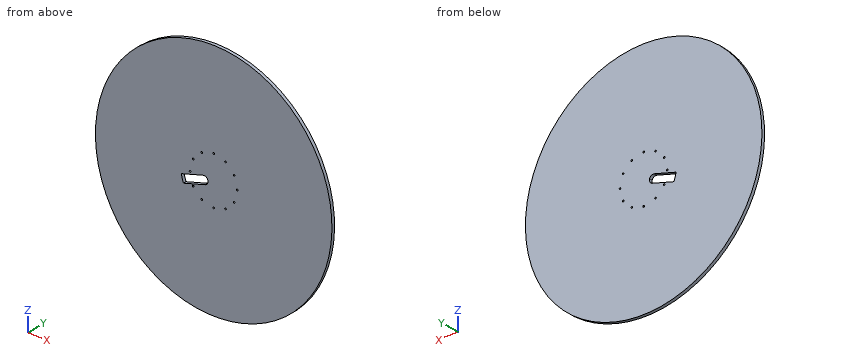
```python
from build123d import *

# Parameters (mm, degrees)
SKETCH1_R           = 300
SKETCH1_R_2         = 2.05
BOSS_EXTRUDE1_DEPTH = 8
CUT_EXTRUDE1_DEPTH  = 425.339486732
FILLET1_R           = 10


with BuildPart() as part:
    # Sketch1 → Boss-Extrude1 (new body)
    with BuildSketch(Plane(origin=(0, 0, 0), x_dir=(1, 0, 0), z_dir=(0, 1, 0))):
        with Locations(Location((0, 0, 0), (0, 0, 270))):
            Circle(SKETCH1_R)
        with Locations(Location((0, 60, 0), (0, 0, 270))):
            Circle(SKETCH1_R_2, mode=Mode.SUBTRACT)
        with Locations(Location((30, 51.961524227, 0), (0, 0, 270))):
            Circle(SKETCH1_R_2, mode=Mode.SUBTRACT)
        with Locations(Location((51.961524227, 30, 0), (0, 0, 270))):
            Circle(SKETCH1_R_2, mode=Mode.SUBTRACT)
        with Locations(Location((60, 0, 0), (0, 0, 270))):
            Circle(SKETCH1_R_2, mode=Mode.SUBTRACT)
        with Locations(Location((51.961524227, -30, 0), (0, 0, 270))):
            Circle(SKETCH1_R_2, mode=Mode.SUBTRACT)
        with Locations(Location((30, -51.961524227, 0), (0, 0, 270))):
            Circle(SKETCH1_R_2, mode=Mode.SUBTRACT)
        with Locations(Location((0, -60, 0), (0, 0, 270))):
            Circle(SKETCH1_R_2, mode=Mode.SUBTRACT)
        with Locations(Location((-30, -51.961524227, 0), (0, 0, 270))):
            Circle(SKETCH1_R_2, mode=Mode.SUBTRACT)
        with Locations(Location((-51.961524227, -30, 0), (0, 0, 270))):
            Circle(SKETCH1_R_2, mode=Mode.SUBTRACT)
        with Locations(Location((-60, 0, 0), (0, 0, 270))):
            Circle(SKETCH1_R_2, mode=Mode.SUBTRACT)
        with Locations(Location((-51.961524227, 30, 0), (0, 0, 270))):
            Circle(SKETCH1_R_2, mode=Mode.SUBTRACT)
        with Locations(Location((-30, 51.961524227, 0), (0, 0, 270))):
            Circle(SKETCH1_R_2, mode=Mode.SUBTRACT)
    extrude(amount=BOSS_EXTRUDE1_DEPTH)

    # Sketch2 → Cut-Extrude1 (cut, through all)
    with BuildSketch(Plane(origin=(0, 8, 0), x_dir=(1, 0, 0), z_dir=(0, 1, 0))):
        with BuildLine():
            Line((-17.622435747, -5.449748467), (-82.039644988, 12.589545274))
            ThreePointArc((-82.039644988, 12.589545274), (-79.925216211, 22.38213157), (-76.646360273, 31.848633518))
            Line((-76.646360273, 31.848633518), (-12.229151031, 13.809339776))
            Line((-12.229151031, 13.809339776), (-17.622435747, -5.449748467))
        make_face()
    extrude(amount=-CUT_EXTRUDE1_DEPTH, mode=Mode.SUBTRACT)

    # Fillet1
    fillet1_edges = [part.edges().sort_by_distance(p)[0] for p in [
        (-17.622435747, 4, 5.449748467),
        (-12.229151031, 4, -13.809339776),
    ]]
    fillet(fillet1_edges, radius=FILLET1_R - 0.0001)  # a hair under: the kernel refuses the full size


solid = part.part
```
Model file for the job. Use its own axes, mm. Give positions to 0.01 mm unless a question says otherwise; leave off trailing zeros. Loops run counter-clockwise (first coordinate to the right, second up) from the corner with the lowest first, then second, coordinate; pieces in that order, holes last. Notation, with made-up numbers: (-22, 57) - (-16, 57) arc R20 cw to (-16, 75) - close; hole circle Ø1 at (51.5, 79.5). An arc over 180 degrees is marked (long way). One line per item, written item: value. Start each with the question number.
1. Slice it at B-B (x = -246). List the corners of the cut face in (y, z).
2. Slice it at A-A (y = 2.25). Give the number of separate pieces and of enclosed holes in the cut face, plus the area to 3 significant figures.
3. Slice it at C-C (z = -185.5). List the corners of the cut face in (x, y).
4. Probe L1, parallel to Z at x = -63, y = 3.75; L2, parallel to X at y = 4.75, z = 60; L3, parallel to Z at x = -76, y = 6. List the from-to ranges inside material, lowest first. Write a range as from..to.
5. Pin check, flat tips, straight feed: pin 1 (3.5 mm diameter, centred on x = -51.96, z = 30, fed in from -Y); pin 2 (3 mm diameter, centred on y = 1.5, z = -39, fed in from +X); pin 3 (3 mm diameter, centred on y = 3.5, z = 101.5, fed in from +X); pin 4 (3 mm diameter, centred on y = 5, z = -216, fed in from +X). Stop position of each tip, or through.
Solution:
1. outline: (0, -171.71) - (8, -171.71) - (8, 171.71) - (0, 171.71) - close
2. separate pieces: 1
2. enclosed holes: 13
2. area: 281,000 mm^2
3. outline: (-235.77, 0) - (235.77, 0) - (235.77, 8) - (-235.77, 8) - close
4. L1: z = -293.31..-28.03, -7.26..293.31
4. L2: x = -293.94..-2.05, 2.05..293.94
4. L3: z = -290.21..-31.67, -10.9..290.21
5. pin 1: passes through
5. pin 2: stops at x = 297.65
5. pin 3: stops at x = 282.84
5. pin 4: stops at x = 209.74
